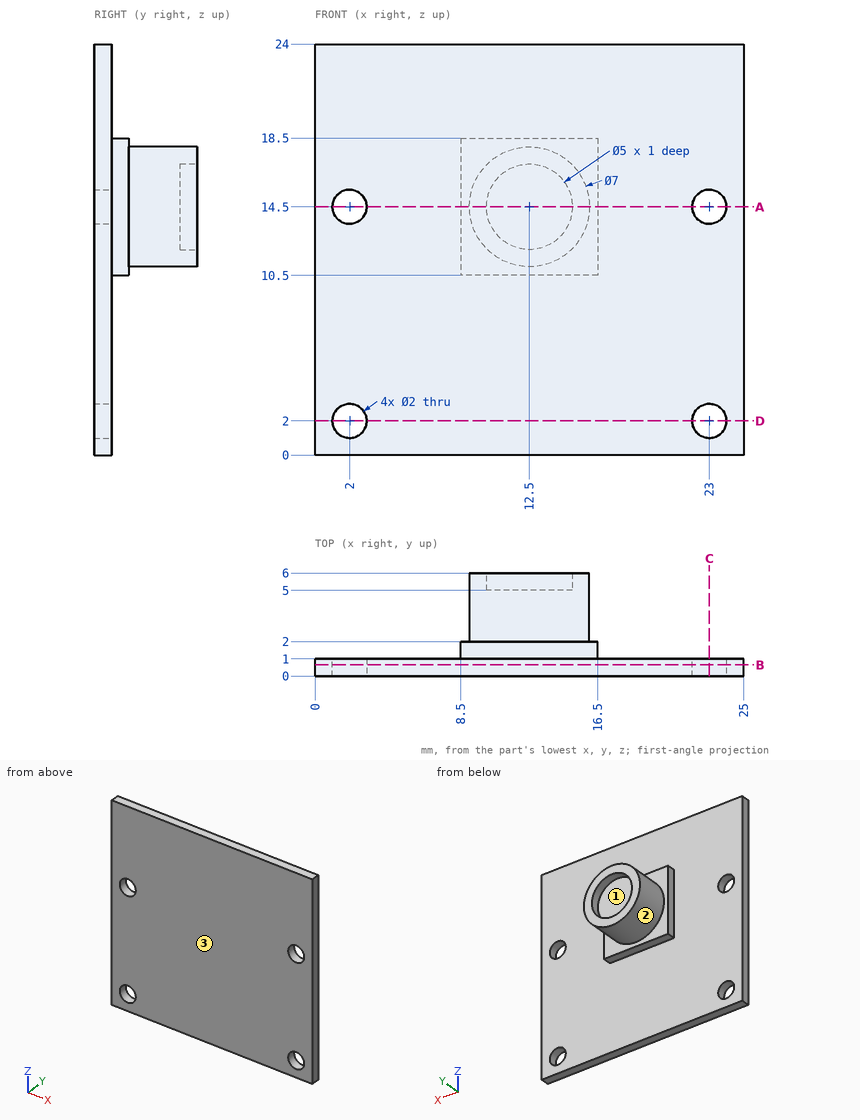
Input: dimensioned drawing with shaded views. Units: mm. Origin: part minimum x, y, z. Coordinates: 2 decimals unless noted, no trailing zeros. Write each loop counter-clockwise with the first axis right and the second up, starting at its lowest first coordinate (ties: lowest second). Pieces come first, ordered by that corner, then holes. Notation, with made-up numbers: (54.25, 12) -> (94.25, 12) arc R29 cw to (94.25, 51) -> close; hole circle Ø3 at (-1, 76.25). An arc over 180 degrees is marked (long way). Return JSON: item names as keys, results as strings. Group by question number.
1) Mould query, pull axis Z, two halves, no side actions, for the marked faces 1, 2 and 3. Classes: +Z half, -Z half, draft (parallel to the pull), parting line (faces both ways), or undercut.
2) Section query D-D, the plane z = 2. Return loops of the section in (x, y), plus the area to 3 significant figures.
3) Section query C-C, the plane x = 23. Return loops of the section in (y, z), plus the area to 3 significant figures.
4) Section query A-A, the plane z = 14.5. Return loops of the section in (x, y), plus the area to 3 significant figures.
5) Ray query, line 1 along X through (y, z) = (0.35, 14.5); line 2 along Z through (x, y) = (2, 0.5); line 3 along X through (y, z) = (5.4, 14.5). Return the intervals inside material, ascending.
6) Section query B-B, the plane y = 0.65. Return loops of the section in (x, z), plus the area to 3 significant figures.
7) Contact query for flat-ended pins moving along their axis: P1, Ø2, axis at x = 20.5, z = 20, coming from the +Y side; P2, Ø1.6, axis at x = 2, z = 2, coming from the +Y side; P3, Ø0.8, axis at y = 1.5, z = 16.5, coming from the +X side; P4, Ø0.5, axis at y = 1.5, z = 13.5, coming from the -X side. Output: stop coordinate, or through.
From the geometry:
{
 "1": {"face 1": "undercut", "face 2": "parting line", "face 3": "draft"},
 "2": {"outline": "(0, 0) -> (1, 0) -> (1, 1) -> (0, 1) -> close; (3, 0) -> (22, 0) -> (22, 1) -> (3, 1) -> close; (24, 0) -> (25, 0) -> (25, 1) -> (24, 1) -> close", "area": "21.0 mm²"},
 "3": {"outline": "(0, 0) -> (1, 0) -> (1, 1) -> (0, 1) -> close; (0, 3) -> (1, 3) -> (1, 13.5) -> (0, 13.5) -> close; (0, 15.5) -> (1, 15.5) -> (1, 24) -> (0, 24) -> close", "area": "20.0 mm²"},
 "4": {"outline": "(0, 0) -> (1, 0) -> (1, 1) -> (0, 1) -> close; (3, 0) -> (22, 0) -> (22, 1) -> (16.5, 1) -> (16.5, 2) -> (16, 2) -> (16, 6) -> (15, 6) -> (15, 5) -> (10, 5) -> (10, 6) -> (9, 6) -> (9, 2) -> (8.5, 2) -> (8.5, 1) -> (3, 1) -> close; (24, 0) -> (25, 0) -> (25, 1) -> (24, 1) -> close", "area": "52.0 mm²"},
 "5": {"line 1": "0 to 1, 3 to 22, 24 to 25", "line 2": "0 to 1, 3 to 13.5, 15.5 to 24", "line 3": "9 to 10, 15 to 16"},
 "6": {"outline": "(0, 0) -> (25, 0) -> (25, 24) -> (0, 24) -> close; hole circle Ø2 at (2, 2); hole circle Ø2 at (2, 14.5); hole circle Ø2 at (23, 2); hole circle Ø2 at (23, 14.5)", "area": "587 mm²"},
 "7": {"P1": "y = 1", "P2": "through", "P3": "x = 16.5", "P4": "x = 8.5"}
}
